Design review of the part built by this model. Coordinates are the model's own, in mm. Face numbers are marked on the shaded views. Coordinates: 2 decimals unless noted, no trailing zeros. Loops run counter-clockwise (first coordinate to the right, second up) from the corner with the lowest first, then second, coordinate; pieces in that order, holes last. Notation, with made-up numbers: M 80,12 L 118,12 A29 cw 118,46 Z; hole C 39.5,-30.75 d3. An arc over 180 degrees is marked long. One line per item, written item: value.
```python
from build123d import *

# Parameters (mm, degrees)
BOSS_EXTRUDE1_DEPTH   = 1.6
SKETCH2_R             = 3.45
BOSS_EXTRUDE2_DEPTH   = 1.4
M5X0_8_TAPPED_HOLE1_D = 4.2


with BuildPart() as part:
    # Sketch1 → Boss-Extrude1 (new body)
    with BuildSketch(Plane.XY):
        with BuildLine():
            Line((3.5, -37.5), (-3.5, -37.5))
            ThreePointArc((-3.5, -37.5), (-4.560660172, -37.060660172), (-5, -36))
            Line((-5, -36), (-5, 36))
            ThreePointArc((-5, 36), (-4.560660172, 37.060660172), (-3.5, 37.5))
            Line((-3.5, 37.5), (3.5, 37.5))
            ThreePointArc((3.5, 37.5), (4.560660172, 37.060660172), (5, 36))
            Line((5, 36), (5, -36))
            ThreePointArc((5, -36), (4.560660172, -37.060660172), (3.5, -37.5))
        make_face()
    extrude(amount=BOSS_EXTRUDE1_DEPTH)

    # Sketch2 → Boss-Extrude2 (add)
    with BuildSketch(Plane.XY.offset(1.6)):
        with Locations((0, 10)):
            Circle(SKETCH2_R)
        with Locations((0, 30)):
            Circle(SKETCH2_R)
        with Locations((0, -10)):
            Circle(SKETCH2_R)
        with Locations((0, -30)):
            Circle(SKETCH2_R)
    extrude(amount=BOSS_EXTRUDE2_DEPTH)

    # M5x0.8 Tapped Hole1 (through all)
    with Locations(Plane.XY.offset(3)):
        with Locations((0, 30), (0, 10), (0, -10), (0, -30)):
            Hole(M5X0_8_TAPPED_HOLE1_D / 2)


solid = part.part
```
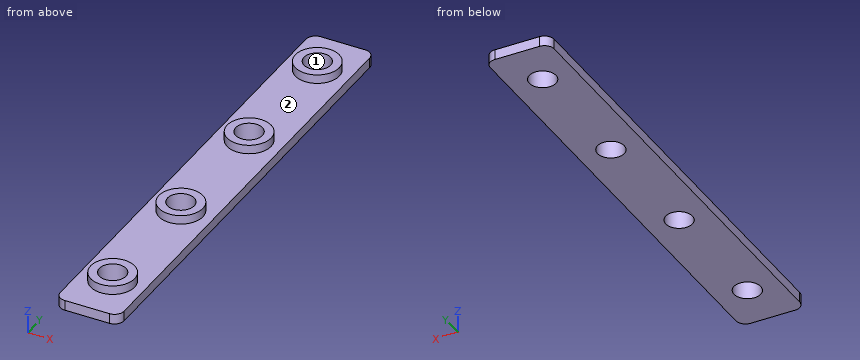
(1) Mouldability with a two-part tool opening along X and no side actions: class the marked faces 1 and 2 as released by +X, released by -X, zero draft, split by the parting line, or undercut.
Reply:
face 1: undercut
face 2: zero draft
(2) We need section D-D on y = 11. State the section outline as (x, z) points, then the cut area to 3 significant figures.
Reply:
outline: M -5,0 L -1.85,0 L -1.85,3 L -3.3,3 L -3.3,1.6 L -5,1.6 Z; M 1.85,0 L 5,0 L 5,1.6 L 3.3,1.6 L 3.3,3 L 1.85,3 Z
area: 14.2 mm2
(3) We need section A-A on z = 2.45. State the section outline as (x, y) points.
Reply:
outline: C 0,-30 d6.9; C 0,-10 d6.9; C 0,10 d6.9; C 0,30 d6.9; hole C 0,-30 d4.2; hole C 0,-10 d4.2; hole C 0,10 d4.2; hole C 0,30 d4.2
(4) We need section B-B on y = -10. State the section outline as (x, z) points.
Reply:
outline: M -5,0 L -2.1,0 L -2.1,3 L -3.45,3 L -3.45,1.6 L -5,1.6 Z; M 2.1,0 L 5,0 L 5,1.6 L 3.45,1.6 L 3.45,3 L 2.1,3 Z
(5) We need section C-C on x = 0. State how many separate pieces and enclosed holes the cut face has, then the cut area to 3 significant figures.
Reply:
separate pieces: 5
enclosed holes: 0
area: 108 mm2
(6) To check wall thickness, follow line 1 along Y through (x, z) = (0, 1); line 2 along Y through (x, z) = (1.5, 1.4); line 3 along Y through (x, z) = (2.75, 2.75). State the ranges of each line that lie inside material, in increasing order. Write a range as [from, to].
Reply:
line 1: y = [-37.5, -32.1], [-27.9, -12.1], [-7.9, 7.9], [12.1, 27.9], [32.1, 37.5]
line 2: y = [-37.5, -31.47], [-28.53, -11.47], [-8.53, 8.53], [11.47, 28.53], [31.47, 37.5]
line 3: y = [-32.08, -27.92], [-12.08, -7.92], [7.92, 12.08], [27.92, 32.08]
